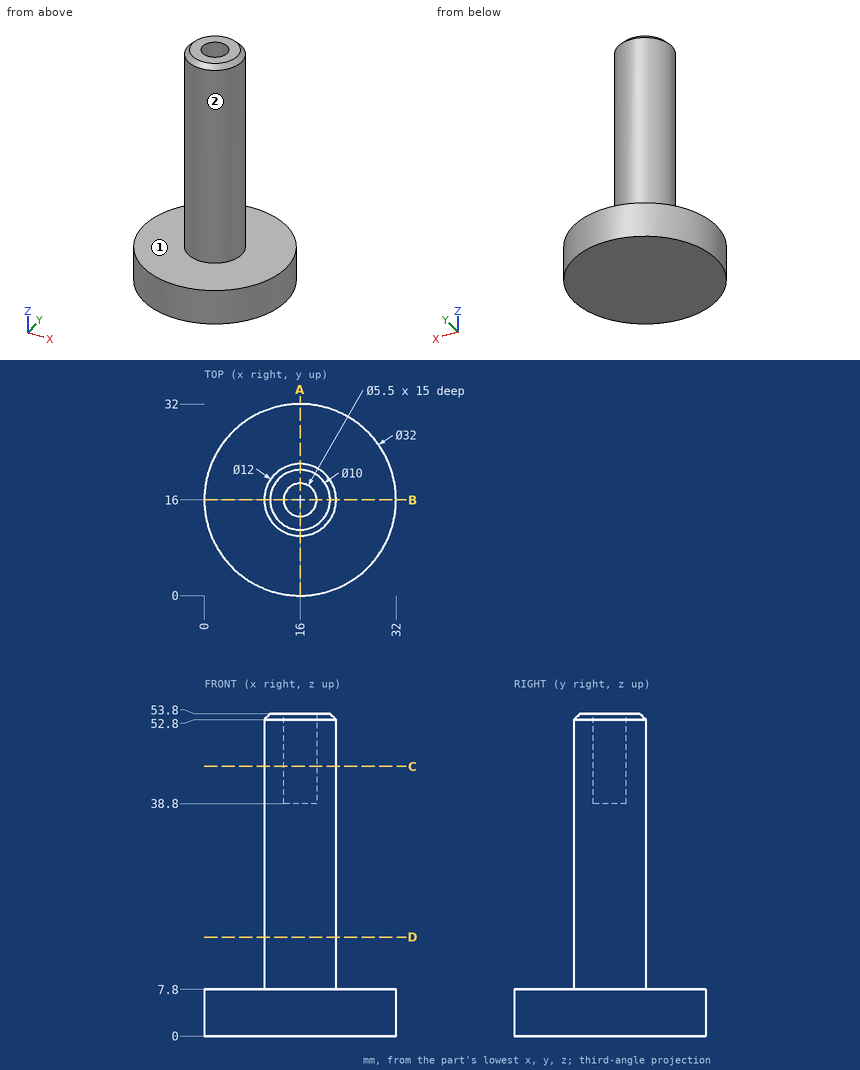
Print and shaded views of the part. All mm, measured from the part's lowest x, y and z. Coordinates: 2 decimals unless noted, no trailing zeros. Loops run counter-clockwise (first coordinate to the right, second up) from the corner with the lowest first, then second, coordinate; pieces in that order, holes last. Notation, with made-up numbers: M -27.75,12 L 11.25,12 A30 cw 11.25,35 Z; hole C 11,25 d8. An arc over 180 degrees is marked long. Use a Markdown table: item, result. Add a question column.
Q1. Cut at D-D (z = 16.5). Write the cut outline in (x, y).
Q2. Mould opens along Y. For the marked faces 1 and 2 say: +Y half, -Y half, draft (parallel to the pull), parting line (faces both ways), or undercut.
Q3. Cut at C-C (z = 45). Write the cut outline in (x, y).
Q4. Probe L1, parallel to Y at x = 16, z = 44; L2, parallel to Z at x = 5, y = 8.5; L3, parallel to X at y = 13.5, z = 39. List the from-to ranges inside material, lowest first.
Q5. Pin check, flat tips, straight feed: P1, Ø2, axis at y = 16, z = 25.5, coming from the +X side; P2, Ø4, axis at x = 16.5, y = 17.5, coming from the -Z side; P3, Ø3, axis at y = 19.5, z = 45, coming from the -X side; P4, Ø8, axis at x = 4, y = 10.5, coming from the +Z side. Stop position of each tip, or through.
Q6. Cut at A-A (x = 16). Write the cut outline in (y, z), and give its area (3 significant figures).
Worked out:
| question | item | result |
|---|---|---|
| 1 | outline | C 16,16 d12 |
| 2 | face 1 | draft |
| 2 | face 2 | parting line |
| 3 | outline | C 16,16 d12; hole C 16,16 d5.5 |
| 4 | L1 | y = 10 to 13.25, 18.75 to 22 |
| 4 | L2 | z = 0 to 7.8 |
| 4 | L3 | x = 10.55 to 14.85, 17.15 to 21.45 |
| 5 | P1 | stops at x = 22 |
| 5 | P2 | stops at z = 0 |
| 5 | P3 | stops at x = 10.34 |
| 5 | P4 | stops at z = 7.8 |
| 6 | outline | M 0,0 L 32,0 L 32,7.8 L 22,7.8 L 22,52.8 L 21,53.8 L 18.75,53.8 L 18.75,38.8 L 13.25,38.8 L 13.25,53.8 L 11,53.8 L 10,52.8 L 10,7.8 L 0,7.8 Z |
| 6 | area | 718 mm2 |
